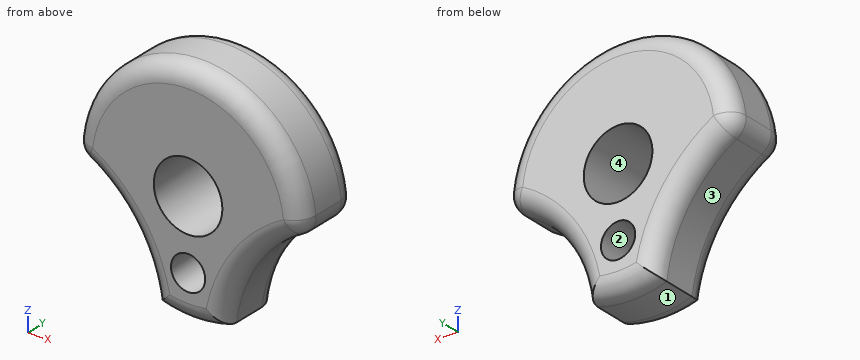
```python
from build123d import *

# Parameters (mm, degrees)
BOSS_EXTRUDE1_DEPTH = 9.525
SKETCH2_R           = 4.7625
SKETCH2_R_2         = 2.3749
CUT_EXTRUDE1_DEPTH  = 10.525
FILLET4_R           = 2.54


with BuildPart() as part:
    # Sketch1 → Boss-Extrude1 (new body)
    with BuildSketch(Plane(origin=(0, 0, 0), x_dir=(1, 0, 0), z_dir=(0, 1, 0))):
        with BuildLine():
            ThreePointArc((-4.7752, 15.139785004), (-8.330712377, 6.107698439), (-15.875, 0))
            ThreePointArc((-15.875, 0), (0, -15.875), (15.875, 0))
            ThreePointArc((15.875, 0), (8.330712377, 6.107698439), (4.7752, 15.139785004))
            ThreePointArc((4.7752, 15.139785004), (0, 15.875), (-4.7752, 15.139785004))
        make_face()
    extrude(amount=BOSS_EXTRUDE1_DEPTH)

    # Sketch2 → Cut-Extrude1 (cut, through all)
    with BuildSketch(Plane(origin=(0, 9.525, 0), x_dir=(1, 0, 0), z_dir=(0, 1, 0))):
        Circle(SKETCH2_R)
        with Locations((0, 9.525)):
            Circle(SKETCH2_R_2)
    extrude(amount=-CUT_EXTRUDE1_DEPTH, mode=Mode.SUBTRACT)

    # Fillet4
    fillet4_edges = [part.edges().sort_by_distance(p)[0] for p in [
        (0, 9.525, 15.875),
        (8.330712377, 9.525, -6.107698439),
        (0, 9.525, -15.875),
        (8.330712377, 0, -6.107698439),
        (0, 0, 15.875),
        (-8.330712377, 0, -6.107698439),
        (0, 0, -15.875),
        (15.875, 4.7625, 0),
        (-15.875, 4.7625, 0),
        (-8.330712377, 9.525, -6.107698439),
    ]]
    fillet(fillet4_edges, radius=FILLET4_R)


solid = part.part
```
Verification items for the finished model (mm, model axes). Face numbers are marked on the shaded views. Coordinates: 2 decimals unless noted, no trailing zeros. Order: outer loops, then holes, each group sorted by start corner. A loop starts at its lowest first (then second) coordinate and runs counter-clockwise, first axis right, second up. Notation, with made-up numbers: (73, 5.5) -> (112, 5.5) arc R22 ccw to (112, 36.5) -> close; hole circle Ø4 at (89, 83.5). An arc over 180 degrees is marked (long way). Put each result on its own line as item: value. Start each with the question number.
1) Material ranges on L1, parallel to Z at x = 0, y = 4 (1 decimal); L2, parallel to Z at x = -2, y = 8.75; L3, parallel to X at y = 9, z = -3.5, recorded low to high.
2) Release check for a two-part mould opening along X. For the marked faces 1, 2, 3 and 4 record: pulls with the +X half, pulls with the -X half, needs draft (parallel to the pull), parting line crosses it, or undercut.
3) Go/stop test with flat-tipped pins: pin 1 (1.5 mm diameter, centred on x = -7, y = 4, fed in from -Z); pin 2 (4 mm diameter, centred on y = 2.5, z = -10, fed in from -X); pin 3 (1 mm diameter, centred on y = 2.5, z = -1.5, fed in from -X). Record where each tip stops, or that it passes through.
4) Cross-section at B-B (y = 5.5). State how many separate pieces and enclosed holes the cut face has, plus the area to 3 significant figures.
5) Cross-section at A-A (x = 0). Enter the section's corners in (y, z) (1 decimal).
Geometry check:
1. L1: z = -15.9 to -11.9, -7.2 to -4.8, 4.8 to 15.9
1. L2: z = -15.03 to -10.81, -8.24 to -4.32, 4.32 to 15.03
1. L3: x = -9.23 to -3.23, 3.23 to 9.23
2. face 1: parting line crosses it
2. face 2: undercut
2. face 3: pulls with the -X half
2. face 4: undercut
3. pin 1: stops at z = -9.72
3. pin 2: stops at x = -7.11
3. pin 3: stops at x = -13.95
4. separate pieces: 1
4. enclosed holes: 2
4. area: 560 mm^2
5. outline: (0, -13.3) arc R2.5 ccw to (2.5, -15.9) -> (7, -15.9) arc R2.5 ccw to (9.5, -13.3) -> (9.5, -11.9) -> (0, -11.9) -> close; (0, -7.2) -> (9.5, -7.2) -> (9.5, -4.8) -> (0, -4.8) -> close; (0, 4.8) -> (9.5, 4.8) -> (9.5, 13.3) arc R2.5 ccw to (7, 15.9) -> (2.5, 15.9) arc R2.5 ccw to (0, 13.3) -> close
